For this review, take the finished solid that the model builds, in its own axes (mm). A direction names the side the tool comes from. Coordinates: 2 decimals unless noted, no trailing zeros. Loops run counter-clockwise (first coordinate to the right, second up) from the corner with the lowest first, then second, coordinate; pieces in that order, holes last. Notation, with made-up numbers: M 71,-3 L 80,-3 A18 ccw 80,28 Z; hole C 78,-6 d4. An arc over 180 degrees is marked long. Use one line per item in the form item = value.
```python
from build123d import *

# Parameters (mm, degrees)
F0_R     = 12
F0_R_2   = 10.85
F0_R_3   = 9.35
F0_R_4   = 6
F1_DEPTH = 5
F2_DEPTH = 70
F3_R     = 10.85
F3_R_2   = 4
F4_DEPTH = 3


with BuildPart() as f1:
    # F0 (on Front) → F1 (new body)
    with BuildSketch(Plane.XZ):
        Circle(F0_R)
        Circle(F0_R_2, mode=Mode.SUBTRACT)
        Circle(F0_R_2)
        Circle(F0_R_3, mode=Mode.SUBTRACT)
        Circle(F0_R_3)
        Circle(F0_R_4, mode=Mode.SUBTRACT)
    extrude(amount=F1_DEPTH)

    # F0 (on Front) → F2 (join)
    with BuildSketch(Plane.XZ):
        Circle(F0_R_2)
        Circle(F0_R_3, mode=Mode.SUBTRACT)
    extrude(amount=-F2_DEPTH)

    # F3 (on face) → F4 (join)
    with BuildSketch(Plane(origin=(0, 70, 0), x_dir=(-1, 0, 0), z_dir=(0, 1, 0))):
        Circle(F3_R)
        Circle(F3_R_2, mode=Mode.SUBTRACT)
    extrude(amount=F4_DEPTH)


solid = f1.part
```
1. Consider section D-D on x = -6.75. Write out the cut boundary in (y, z).
Computed values:
outline = M -5,-9.92 L 0,-9.92 L 0,-8.49 L 73,-8.49 L 73,8.49 L 0,8.49 L 0,9.92 L -5,9.92 Z; hole M 0,-6.47 L 70,-6.47 L 70,6.47 L 0,6.47 Z
2. Tool access review of faces 1 (the face through (0.867, 71.479, -3.905)), 2 (the face through (-2, 70, -4)), 3 (the face through (-6, -2, 0)), 4 (the face through (-3, 0, -11)): name each direction out of +Z, -Z, +X, -X, +Y, -Y from which nothing blocks a thin tool from reaching the whole face with its end or side.
Computed values:
face_1 = +Y, -Y
face_2 = none
face_3 = -Y
face_4 = +Y
3. Wall thickness on line 1 along X through (y, z) = (41, 0.25); line 2 along Y through (x, z) = (-4.75, -6); line 3 along Z through (x, y) = (0, 70.95): over which ranges is each line inside the solid? List them lowest first. Write a range as from..to.
Computed values:
line_1 = -10.85..-9.35, 9.35..10.85
line_2 = -5..0, 70..73
line_3 = -10.85..-4, 4..10.85
4. Consider section C-C on y = 4. Write out the cut boundary in (x, z).
Computed values:
outline = C 0,0 d21.7; hole C 0,0 d18.7
5. Consider section A-A on z = 0. Write out the cut boundary in (x, y), plus the area to 3 significant figures.
Computed values:
outline = M -12,-5 L -6,-5 L -6,0 L -9.35,0 L -9.35,70 L -4,70 L -4,73 L -10.85,73 L -10.85,0 L -12,0 Z; M 4,70 L 9.35,70 L 9.35,0 L 6,0 L 6,-5 L 12,-5 L 12,0 L 10.85,0 L 10.85,73 L 4,73 Z
area = 311 mm2
6. Draft analysis for pull direction Z (two halves, no side actions). For faces 5 (the face through (6, 0, -2)), 6 (the face through (-11.99, -2.46, 0.53)), 7 (the face through (-5, 73, 0)), state which applies: +Z half, -Z half, draft (parallel to the pull), parting line (faces both ways), or undercut.
Computed values:
face_5 = undercut
face_6 = parting line
face_7 = draft
7. Consider section B-B on x = 0. Write out the cut boundary in (y, z).
Computed values:
outline = M -5,-12 L 0,-12 L 0,-10.85 L 73,-10.85 L 73,-4 L 70,-4 L 70,-9.35 L 0,-9.35 L 0,-6 L -5,-6 Z; M -5,6 L 0,6 L 0,9.35 L 70,9.35 L 70,4 L 73,4 L 73,10.85 L 0,10.85 L 0,12 L -5,12 Z
8. For pin 1 Ø5 at (x, y) = (-3, 63.5) entering from -Z; pin 2 Ø5 at (x, y) = (8.5, 45.5) entering from +Z; pin 3 Ø12 at (y, z) = (41.5, 6) entering from -X; pin 4 Ø13 at (x, z) = (0, 0) entering from -Y, all flat-tipped, find the tip position at first contact; note any pin that passes through.
Computed values:
pin_1 = -10.84
pin_2 = 9.04
pin_3 = -10.85
pin_4 = -5
